Part model, mm, in its own coordinate system. Give positions to 0.01 mm unless a question says otherwise; leave off trailing zeros. Order: outer loops, then holes, each group sorted by start corner. A loop starts at its lowest first (then second) coordinate and runs counter-clockwise, first axis right, second up. Notation, with made-up numbers: M 19,27 L 39,27 A4 cw 39,34 Z; hole C -22,38.25 d11. An arc over 180 degrees is marked long. Answer as a JSON object with one key per item and string values.
from build123d import *

# Parameters (mm, degrees)
BASE_FLANGE1_DEPTH         = 5
F_5_2_5_2_DIAMETER_HOLE1_D = 5.2
F_7_1_7_1_DIAMETER_HOLE1_D = 7.1
F_6_5_6_5_DIAMETER_HOLE1_D = 6.5
F_4_2_4_2_DIAMETER_HOLE1_D = 4.2


# Sheet-metal steps are written as plain solids
with BuildPart() as part:
    # Sketch7 → Base-Flange1 (new body)
    with BuildSketch(Plane.XY.offset(5)):
        with BuildLine():
            Line((-30, -147.320508076), (-30, -150))
            ThreePointArc((-30, -150), (-27.071067812, -157.071067812), (-20, -160))
            Line((-20, -160), (20, -160))
            ThreePointArc((20, -160), (29.659258263, -152.588190451), (25, -141.339745962))
            ThreePointArc((25, -141.339745962), (21.339745962, -137.679491924), (20, -132.679491924))
            Line((20, -132.679491924), (20, -61))
            ThreePointArc((20, -61), (21.464466094, -57.464466094), (25, -56))
            Line((25, -56), (26.5, -56))
            ThreePointArc((26.5, -56), (30.291825885, -55.253218708), (33.517318844, -53.124411291))
            ThreePointArc((33.517318844, -53.124411291), (35.066201479, -52.086695747), (36.887562932, -51.688533184))
            ThreePointArc((36.887562932, -51.688533184), (50.4004845, -39.360191171), (40.184210526, -24.187359787))
            ThreePointArc((40.184210526, -24.187359787), (37.526402929, -22.398480791), (36.5, -19.363595898))
            Line((36.5, -19.363595898), (36.5, 11.495546893))
            Line((36.5, 11.495546893), (107.655738061, 102.897284867))
            ThreePointArc((107.655738061, 102.897284867), (111.029837924, 100.693170117), (115, 100))
            ThreePointArc((115, 100), (122.071067812, 102.928932188), (125, 110))
            Line((125, 110), (125, 150))
            ThreePointArc((125, 150), (122.071067812, 157.071067812), (115, 160))
            Line((115, 160), (109.8448211, 160))
            ThreePointArc((109.8448211, 160), (105.484755829, 158.999435028), (101.997196274, 156.197966166))
            Line((101.997196274, 156.197966166), (20.637667976, 53.183681001))
            ThreePointArc((20.637667976, 53.183681001), (17.310502968, 50.830398319), (13.320715378, 50))
            Line((13.320715378, 50), (-12.442983516, 50))
            ThreePointArc((-12.442983516, 50), (-15.658335228, 50.531023637), (-18.532201388, 52.067697326))
            Line((-18.532201388, 52.067697326), (-101.997626249, 156.252326096))
            ThreePointArc((-101.997626249, 156.252326096), (-105.473226973, 159.014523308), (-109.802010811, 160))
            Line((-109.802010811, 160), (-115, 160))
            ThreePointArc((-115, 160), (-122.071067812, 157.071067812), (-125, 150))
            Line((-125, 150), (-125, 110))
            ThreePointArc((-125, 110), (-119.472924821, 101.056122567), (-109.001411291, 101.998941726))
            Line((-109.001411291, 101.998941726), (-36.5, 11.5))
            Line((-36.5, 11.5), (-36.5, -19.363595898))
            ThreePointArc((-36.5, -19.363595898), (-37.526402929, -22.398480791), (-40.184210526, -24.187359787))
            ThreePointArc((-40.184210526, -24.187359787), (-50.4004845, -39.360191171), (-36.887562932, -51.688533184))
            ThreePointArc((-36.887562932, -51.688533184), (-35.066201479, -52.086695747), (-33.517318844, -53.124411291))
            ThreePointArc((-33.517318844, -53.124411291), (-30.291825885, -55.253218708), (-26.5, -56))
            Line((-26.5, -56), (-25, -56))
            ThreePointArc((-25, -56), (-21.464466094, -57.464466094), (-20, -61))
            Line((-20, -61), (-20, -130))
            ThreePointArc((-20, -130), (-21.339745962, -135), (-25, -138.660254038))
            ThreePointArc((-25, -138.660254038), (-28.660254038, -142.320508076), (-30, -147.320508076))
        make_face()
        with BuildLine():
            Line((117.6, 136.4), (117.6, 129.6))
            ThreePointArc((117.6, 129.6), (115, 127), (112.4, 129.6))
            Line((112.4, 129.6), (112.4, 136.4))
            ThreePointArc((112.4, 136.4), (115, 139), (117.6, 136.4))
        make_face(mode=Mode.SUBTRACT)
        with BuildLine():
            Line((-112.4, 136.4), (-112.4, 129.6))
            ThreePointArc((-112.4, 129.6), (-115, 127), (-117.6, 129.6))
            Line((-117.6, 129.6), (-117.6, 136.4))
            ThreePointArc((-117.6, 136.4), (-115, 139), (-112.4, 136.4))
        make_face(mode=Mode.SUBTRACT)
        with BuildLine():
            Line((2.6, -129.6), (2.6, -136.4))
            ThreePointArc((2.6, -136.4), (0, -139), (-2.6, -136.4))
            Line((-2.6, -136.4), (-2.6, -129.6))
            ThreePointArc((-2.6, -129.6), (0, -127), (2.6, -129.6))
        make_face(mode=Mode.SUBTRACT)
        with BuildLine():
            Line((-20, -36), (-20, 30))
            ThreePointArc((-20, 30), (-18.535533906, 33.535533906), (-15, 35))
            Line((-15, 35), (15, 35))
            ThreePointArc((15, 35), (18.535533906, 33.535533906), (20, 30))
            Line((20, 30), (20, -36))
            ThreePointArc((20, -36), (18.535533906, -39.535533906), (15, -41))
            Line((15, -41), (-15, -41))
            ThreePointArc((-15, -41), (-18.535533906, -39.535533906), (-20, -36))
        make_face(mode=Mode.SUBTRACT)
    extrude(amount=-BASE_FLANGE1_DEPTH)

    # Ø5.2 (5.2) Diameter Hole1 (through all)
    with Locations(Plane.XY.offset(5)):
        with Locations((42.3, -37.693898678), (42.3, 42.306101322)):
            Hole(F_5_2_5_2_DIAMETER_HOLE1_D / 2)

    # Ø7.1 (7.1) Diameter Hole1 (through all)
    with Locations(Plane.XY.offset(5)):
        with Locations((-42.3, -37.693898678), (-42.3, 42.306101322)):
            Hole(F_7_1_7_1_DIAMETER_HOLE1_D / 2)

    # Ø6.5 (6.5) Diameter Hole1 (through all)
    with Locations(Plane.XY.offset(5)):
        with Locations((-30, -43.5), (-30, 43.5), (-30, -27.5), (-30, 27.5), (30, -43.5), (30, -27.5), (30, 27.5), (30, 43.5)):
            Hole(F_6_5_6_5_DIAMETER_HOLE1_D / 2)

    # Ø4.2 (4.2) Diameter Hole1 (through all)
    with Locations(Plane.XY.offset(5)):
        with Locations((0, -150), (-115, 150), (115, 150)):
            Hole(F_4_2_4_2_DIAMETER_HOLE1_D / 2)


solid = part.part
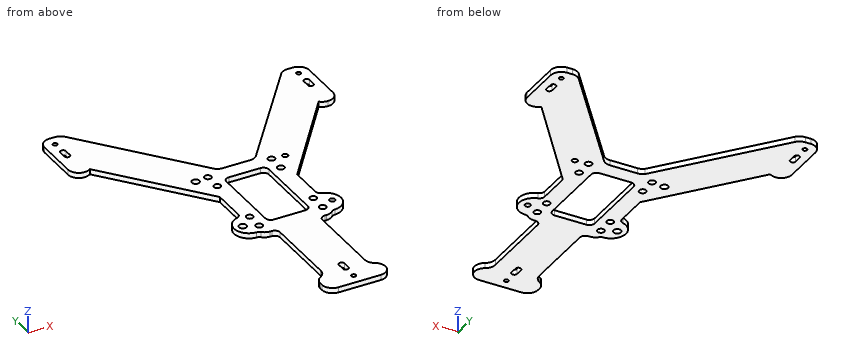
1. Probe line 1 along Y through (x, z) = (-42.3, 2.95); line 2 along Y through (x, z) = (-27.5, 4.65); line 3 along Y through (x, z) = (-43, 3.65). List the from-to ranges inside material, lowest first.
Worked answers:
{"line 1": "y = -50.44 to -41.24, -34.14 to -24.95, 18.74 to 38.76, 45.86 to 81.74", "line 2": "y = -156.61 to -140.71, -55.95 to -45.58, -41.42 to -29.58, -25.42 to 25.42, 29.58 to 41.42, 45.58 to 63.26", "line 3": "y = -50.09 to -41.17, -34.21 to -25.29, 19.61 to 38.83, 45.79 to 82.61"}
2. Pin check, flat tips, straight feed: P1, Ø1, axis at x = 35.5, y = 23.5, coming from the -Z side; P2, Ø1, axis at x = 73.5, z = 4.5, coming from the +Y side. Stop position of each tip, or through.
Worked answers:
{"P1": "stops at z = 0", "P2": "stops at y = 120.75"}
3. Cut at A-A on y = -27.5. Give the cut face in (x, z).
Worked answers:
{"outline": "M -46.1,0 L -33.25,0 L -33.25,5 L -46.1,5 Z; M -26.75,0 L -20,0 L -20,5 L -26.75,5 Z; M 20,0 L 26.75,0 L 26.75,5 L 20,5 Z; M 33.25,0 L 46.1,0 L 46.1,5 L 33.25,5 Z"}
4. Cut at C-C on x = -78. Give the cut face in (y, z), plus the area to 3 significant figures.
Worked answers:
{"outline": "M 63.3,0 L 126.3,0 L 126.3,5 L 63.3,5 Z", "area": "315 mm^2"}
5. Cut at B-B on z = 3.45. State how many separate pieces and enclosed holes the cut face has, plus the area to 3 significant figures.
Worked answers:
{"separate pieces": "1", "enclosed holes": "19", "area": "20,500 mm^2"}
